Build history of the part. All positions in model axes, mm. Face numbers are marked on the shaded views. A direction names the side the tool comes from. Round coordinates to 2 decimals unless told otherwise and drop trailing zeros. Write each loop counter-clockwise with the first axis right and the second up, starting at its lowest first coordinate (ties: lowest second). Pieces come first, ordered by that corner, then holes. Notation, with made-up numbers: (-14, 4.5) - (-7, 4.5) arc R18 ccw to (-7, 21.5) - close; hole circle Ø11 at (26, 22). An arc over 180 degrees is marked (long way). One line per question, with ' | ' between items.
from build123d import *

# Parameters (mm, degrees)
SKETCH1_W             = 20.32
SKETCH1_H             = 40.64
EXTRUDE1_DEPTH        = 25.4
SKETCH2_W             = 20.32
SKETCH2_H             = 40.64
EXTRUDE2_DEPTH        = 2.38125
SKETCH3_W             = 20.32
SKETCH3_H             = 40.64
EXTRUDE3_DEPTH        = 4.445
EXTRUDE4_DEPTH        = 2.38125
SKETCH5_R             = 7.62
EXTRUDE5_DEPTH        = 3.4925
CHAMFER1_SIZE         = 2.54
CHAMFER1_SIZE2        = 1.466469684
EXTRUDE6_DEPTH        = 0.635
SKETCH8_R             = 2.778125
EXTRUDE7_DEPTH        = 3.175
CHAMFER2_SIZE         = 2.54
CHAMFER2_SIZE2        = 1.466469684
CHAMFER2_PART_2_SIZE  = 2.54
CHAMFER2_PART_2_SIZE2 = 1.466469684
FILLET1_R             = 1.016
FILLET2_R             = 1.524
SKETCH9_W             = 6.35
SKETCH9_H             = 2.54
EXTRUDE8_DEPTH        = 2.38125
SKETCH10_W            = 5.08
SKETCH10_H            = 1.27
CUT_EXTRUDE1_DEPTH    = 2.38125


with BuildPart() as part:
    # Sketch1 → Extrude1 (new body)
    with BuildSketch(Plane(origin=(0, 0, 0), x_dir=(1, 0, 0), z_dir=(0, 1, 0))):
        with Locations((0, -10.16)):
            Rectangle(SKETCH1_W, SKETCH1_H)
    extrude(amount=EXTRUDE1_DEPTH)

    # Sketch2 → Extrude2 (add)
    with BuildSketch(Plane(origin=(0, 25.4, 0), x_dir=(-1, 0, 0), z_dir=(0, 1, 0))):
        with Locations((0, 10.16)):
            Rectangle(SKETCH2_W, SKETCH2_H)
        with BuildLine():
            ThreePointArc((6.731, -15.64118631), (5.08, -11.8364), (3.429, -15.64118631))
            Line((3.429, -15.64118631), (3.429, -17.78))
            Line((3.429, -17.78), (-3.429, -17.78))
            Line((-3.429, -17.78), (-3.429, -15.64118631))
            ThreePointArc((-3.429, -15.64118631), (-5.08, -11.8364), (-6.731, -15.64118631))
            Line((-6.731, -15.64118631), (-6.731, -17.78))
            Line((-6.731, -17.78), (-10.16, -17.78))
            Line((-10.16, -17.78), (-10.16, -10.16))
            Line((-10.16, -10.16), (10.16, -10.16))
            Line((10.16, -10.16), (10.16, -17.78))
            Line((10.16, -17.78), (6.731, -17.78))
            Line((6.731, -17.78), (6.731, -15.64118631))
        make_face()
        with BuildLine():
            ThreePointArc((-6.731, 35.70718631), (-5.08, 31.9024), (-3.429, 35.70718631))
            Line((-3.429, 35.70718631), (-3.429, 38.1))
            Line((-3.429, 38.1), (3.429, 38.1))
            Line((3.429, 38.1), (3.429, 35.70718631))
            ThreePointArc((3.429, 35.70718631), (5.08, 31.9024), (6.731, 35.70718631))
            Line((6.731, 35.70718631), (6.731, 38.1))
            Line((6.731, 38.1), (10.16, 38.1))
            Line((10.16, 38.1), (10.16, 30.48))
            Line((10.16, 30.48), (-10.16, 30.48))
            Line((-10.16, 30.48), (-10.16, 38.1))
            Line((-10.16, 38.1), (-6.731, 38.1))
            Line((-6.731, 38.1), (-6.731, 35.70718631))
        make_face()
    extrude(amount=EXTRUDE2_DEPTH)

    # Sketch3 → Extrude3 (add)
    with BuildSketch(Plane(origin=(0, 27.78125, 0), x_dir=(-1, 0, 0), z_dir=(0, 1, 0))):
        with Locations((0, 10.16)):
            Rectangle(SKETCH3_W, SKETCH3_H)
    extrude(amount=EXTRUDE3_DEPTH)

    # Sketch4 → Extrude4 (add)
    with BuildSketch(Plane(origin=(0, 32.22625, 0), x_dir=(-1, 0, 0), z_dir=(0, 1, 0))):
        with BuildLine():
            Line((9.652, 2.228840954), (9.652, 24.13))
            Line((9.652, 24.13), (4.655896906, 24.13))
            ThreePointArc((4.655896906, 24.13), (0, 27.178), (-4.655896906, 24.13))
            Line((-4.655896906, 24.13), (-9.652, 24.13))
            Line((-9.652, 24.13), (-9.652, 2.228840954))
            ThreePointArc((-9.652, 2.228840954), (0, -9.906), (9.652, 2.228840954))
        make_face()
    extrude(amount=EXTRUDE4_DEPTH)

    # Sketch5 → Extrude5 (add)
    with BuildSketch(Plane(origin=(0, 34.6075, 0), x_dir=(-1, 0, 0), z_dir=(0, 1, 0))):
        Circle(SKETCH5_R)
    extrude(amount=EXTRUDE5_DEPTH)

    # Chamfer1
    chamfer1_edges = [part.edges().sort_by_distance(p)[0] for p in [
        (7.62, 38.1, 0),
    ]]
    chamfer1_side = [part.faces().sort_by_distance(p)[0] for p in [
        (0, 38.1, 0),
    ]]
    chamfer(chamfer1_edges, length=CHAMFER1_SIZE, length2=CHAMFER1_SIZE2, reference=chamfer1_side[0])

    # Sketch7 → Extrude6 (add, symmetric)
    with BuildSketch(Plane(origin=(0, 0, 0), x_dir=(0, 0, -1), z_dir=(1, 0, 0))):
        Polygon((15.494, 27.78125), (12.954, 29.55925), (10.16, 29.55925), (10.16, 27.78125), align=None)
    extrude6 = extrude(amount=EXTRUDE6_DEPTH, both=True)

    # Mirror1: Extrude6 across plane
    add(extrude6.mirror(Plane(origin=(0, 0, 10.16), x_dir=(1, 0, 0), z_dir=(0, 0, -1))))

    # Sketch8 → Extrude7 (add)
    with BuildSketch(Plane(origin=(0, 38.1, 0), x_dir=(-1, 0, 0), z_dir=(0, 1, 0))):
        Circle(SKETCH8_R)
    extrude(amount=EXTRUDE7_DEPTH)

    # Chamfer2
    chamfer2_edges = [part.edges().sort_by_distance(p)[0] for p in [
        (0, 0, -10.16),
    ]]
    chamfer2_side = [part.faces().sort_by_distance(p)[0] for p in [
        (0, 12.7, -10.16),
    ]]
    chamfer(chamfer2_edges, length=CHAMFER2_SIZE, length2=CHAMFER2_SIZE2, reference=chamfer2_side[0])

    # Chamfer2 part 2
    chamfer2_part_2_edges = [part.edges().sort_by_distance(p)[0] for p in [
        (0, 0, 30.48),
    ]]
    chamfer2_part_2_side = [part.faces().sort_by_distance(p)[0] for p in [
        (0, 12.7, 30.48),
    ]]
    chamfer(chamfer2_part_2_edges, length=CHAMFER2_PART_2_SIZE, length2=CHAMFER2_PART_2_SIZE2, reference=chamfer2_part_2_side[0])

    # Fillet1
    fillet1_edges = [part.edges().sort_by_distance(p)[0] for p in [
        (-10.16, 30.00375, -10.16),
        (10.16, 30.00375, -10.16),
        (10.16, 30.00375, 30.48),
        (10.16, 0, 10.16),
        (10.16, 1.27, -9.426765158),
        (10.16, 13.97, -10.16),
        (0, 0, -8.693530316),
        (0, 2.54, -10.16),
        (-10.16, 13.97, -10.16),
        (-10.16, 1.27, -9.426765158),
        (10.16, 13.97, 30.48),
        (10.16, 1.27, 29.746765158),
        (0, 2.54, 30.48),
        (-10.16, 0, 10.16),
        (0, 0, 29.013530316),
        (-10.16, 1.27, 29.746765158),
        (-10.16, 13.97, 30.48),
        (-10.16, 30.00375, 30.48),
    ]]
    fillet(fillet1_edges, radius=FILLET1_R)

    # Fillet2
    fillet2_edges = [part.edges().sort_by_distance(p)[0] for p in [
        (-10.16, 26.590625, 38.1),
        (10.16, 26.590625, 38.1),
        (-10.16, 26.590625, -17.78),
        (10.16, 26.590625, -17.78),
    ]]
    fillet(fillet2_edges, radius=FILLET2_R)

    # Sketch9 → Extrude8 (add)
    with BuildSketch(Plane(origin=(0, 0, -10.16), x_dir=(-1, 0, 0), z_dir=(0, 0, -1))):
        with Locations((0, 4.318)):
            Rectangle(SKETCH9_W, SKETCH9_H)
    extrude(amount=EXTRUDE8_DEPTH)

    # Sketch10 → Cut-Extrude1 (cut)
    with BuildSketch(Plane(origin=(0, 0, -12.54125), x_dir=(-1, 0, 0), z_dir=(0, 0, -1))):
        with Locations((0, 4.318)):
            Rectangle(SKETCH10_W, SKETCH10_H)
    extrude(amount=-CUT_EXTRUDE1_DEPTH, mode=Mode.SUBTRACT)


solid = part.part
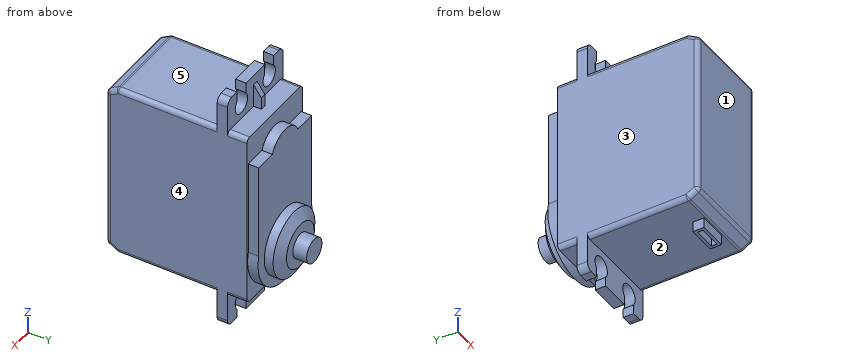
Q1. Saw through at A-A, the plane z = 21.5. List the corners of the cut face in (x, y).
Found:
outline: (-10.16, 1.02) arc R1.02 ccw to (-9.14, 0) - (9.14, 0) arc R1.02 ccw to (10.16, 1.02) - (10.16, 32.23) - (9.65, 32.23) - (9.65, 34.61) - (-9.65, 34.61) - (-9.65, 32.23) - (-10.16, 32.23) - close
Q2. Drop flat-ended pins along their axis: pin 1 (1 mm diameter, centred on y = 4.5, z = -12, fed in from +X) (3 decimals); pin 2 (6 mm diameter, centred on x = -5.5, y = 35, fed in from +Z); pin 3 (0.9 mm diameter, centred on y = 28.5, z = -13.5, fed in from -X) (3 decimals). Give the stop position or say it passes through.
Found:
pin 1: x = 3.175 | pin 2: z = 30.48 | pin 3: x = -0.635
Q3. Saw through at B-B, the plane y = 35.5. List the corners of the cut face in (x, z), then the cut area to 3 significant figures.
Found:
outline: circle Ø15.24 at (0, 0) | area: 182 mm^2
Q4. Drill centre lines: L1, parallel to Y at x = -1.5, z = -12; L2, parallel to Y at x = -0.25, z = 24; L3, parallel to Y at x = -2, z = 33.5. Where is each one in solid material? Low to high. Write a range as from..to.
Found:
L1: 3.05..3.68, 4.95..5.59, 25.4..27.78 | L2: 0..34.61 | L3: 25.4..27.78
Q5. Which spindle directions (+Z, -Z, +X, -X, +Y, -Y) get a long thin tool onto all of the face, cutting with end or side? Do the marked faces 4 and 5. Say none if no direction does.
Found:
face 4: +Z, -Z, +X, +Y, -Y | face 5: +Z, +X, -X, -Y
Q6. Pull direction Y, two halves, no side cores. Call the marked faces 1, 2 and 3: +Y half, -Y half, draft (parallel to the pull), parting line (faces both ways), or undercut.
Found:
face 1: -Y half | face 2: undercut | face 3: draft
